```python
from build123d import *

# Parameters (mm, degrees)
SKETCH_1_R          = 3.6
EXTRUDE_1_DEPTH     = 4
CUT_EXTRUDE_1_DEPTH = 2
SKETCH_3_R          = 1.732050808
SKETCH_4_R          = 1.5
CHAMFER_1_SIZE      = 0.5
CHAMFER_2_SIZE      = 0.2


with BuildPart() as part:
    # 草图1 → 凸台-拉伸1 (new body)
    with BuildSketch(Plane(origin=(0, 0, 0), x_dir=(1, 0, 0), z_dir=(0, 1, 0))):
        with Locations(Location((0, 0, 0), (0, 0, 270))):
            Circle(SKETCH_1_R)
    extrude(amount=EXTRUDE_1_DEPTH)

    # 草图2 → 切除-拉伸1 (cut)
    with BuildSketch(Plane(origin=(0, 4, 0), x_dir=(1, 0, 0), z_dir=(0, 1, 0))):
        Polygon((1.732050808, 0), (0.866025404, 1.5), (-0.866025404, 1.5), (-1.732050808, 0), (-0.866025404, -1.5), (0.866025404, -1.5), align=None)
    extrude(amount=-CUT_EXTRUDE_1_DEPTH, mode=Mode.SUBTRACT)

    # 草图3 → 切除-放样1 section 0
    with BuildSketch(Plane(origin=(0, 4, 0), x_dir=(1, 0, 0), z_dir=(0, 1, 0))):
        Circle(SKETCH_3_R)
    # 草图4 → 切除-放样1 section 1
    with BuildSketch(Plane(origin=(0, 3.7, 0), x_dir=(1, 0, 0), z_dir=(0, 1, 0))):
        Circle(SKETCH_4_R)
    loft(mode=Mode.SUBTRACT)

    # 倒角1
    chamfer_1_edges = [part.edges().sort_by_distance(p)[0] for p in [
        (0, 4, -3.6),
    ]]
    chamfer(chamfer_1_edges, length=CHAMFER_1_SIZE)

    # 倒角2
    chamfer_2_edges = [part.edges().sort_by_distance(p)[0] for p in [
        (0, 0, -3.6),
    ]]
    chamfer(chamfer_2_edges, length=CHAMFER_2_SIZE)


solid = part.part
```
Input: part model. Units: mm. Frame: model coordinates. A direction names the side the tool comes from. Round coordinates to 2 decimals unless told otherwise and drop trailing zeros. Loops run counter-clockwise (first coordinate to the right, second up) from the corner with the lowest first, then second, coordinate; pieces in that order, holes last. Notation, with made-up numbers: (-27, -29.5) -> (19, -29.5) arc R16 cw to (19, -9.5) -> close; hole circle Ø7 at (37.5, 47). An arc over 180 degrees is marked (long way). One line per item, written item: value.
(1) Section D-D (y = 0.5). Return the cut outline in (x, z), plus the area to 3 significant figures.
Geometry check:
outline: circle Ø7.2 at (0, 0)
area: 40.7 mm2
(2) Mould query, pull axis X, two halves, no side actions, for faces 3 (the face through (-1.404, 3.848, 0.797)), 4 (the face through (-1.379, 1.827, 3.325)), 5 (the face through (0, 0, 0)). Classes: pulls with the +X half, pulls with the -X half, needs draft (parallel to the pull), parting line crosses it, or undercut.
Geometry check:
face 3: undercut
face 4: parting line crosses it
face 5: needs draft
(3) Section C-C (y = 3.6). Return the cut outline in (x, z), plus the area to 3 significant figures.
Geometry check:
outline: circle Ø7 at (0, 0); hole (-1.73, 0) -> (-0.87, -1.5) -> (0.87, -1.5) -> (1.73, 0) -> (0.87, 1.5) -> (-0.87, 1.5) -> close
area: 30.7 mm2
(4) Section B-B (x = 0). Return the cut outline in (y, z), plus the area to 3 significant figures.
Geometry check:
outline: (0, -3.4) -> (0.2, -3.6) -> (3.5, -3.6) -> (4, -3.1) -> (4, -1.73) -> (3.7, -1.5) -> (2, -1.5) -> (2, 1.5) -> (3.7, 1.5) -> (4, 1.73) -> (4, 3.1) -> (3.5, 3.6) -> (0.2, 3.6) -> (0, 3.4) -> close
area: 22.4 mm2
(5) Material intervals for line 1 (Y direction, x = 0.25, z = -0.25); line 2 (Z direction, x = -1, y = 2.3); line 3 (X direction, y = 2.45, z = -0.5), sorted ascending. Write a range as [from, to].
Geometry check:
line 1: [0, 2]
line 2: [-3.46, -1.27], [1.27, 3.46]
line 3: [-3.57, -1.44], [1.44, 3.57]
(6) Pin query (flat end, axial travel): pin 1 (2 mm diameter, centred on x = -0.5, z = -0.5, fed in from -Y); pin 2 (2 mm diameter, centred on x = -2, y = 1.5, fed in from +Z); pin 3 (2 mm diameter, centred on y = 0.5, z = 2.5, fed in from -X); pin 4 (1 mm diameter, centred on x = -1, y = 3, fed in from -Z). Return the tip coordinate at first contact, or that it passes through.
Geometry check:
pin 1: y = 0
pin 2: z = 3.46
pin 3: x = -3.27
pin 4: z = -3.57
(7) Section A-A (y = 2.3). Return the cut outline in (x, z), plus the area to 3 significant figures.
Geometry check:
outline: circle Ø7.2 at (0, 0); hole (-1.73, 0) -> (-0.87, -1.5) -> (0.87, -1.5) -> (1.73, 0) -> (0.87, 1.5) -> (-0.87, 1.5) -> close
area: 32.9 mm2
(8) Set-up query: faces 1 (the face through (1.39, 3.85, 0.82)), 2 (the face through (-1.334, 4, 1.334)). Return all of +Z, -Z, +X, -X, +Y, -Y with unobstructed straight access to the full face (end or side cutting, diameter ignored); none if empty.
Geometry check:
face 1: +Y
face 2: +Z, -Z, +X, -X, +Y
